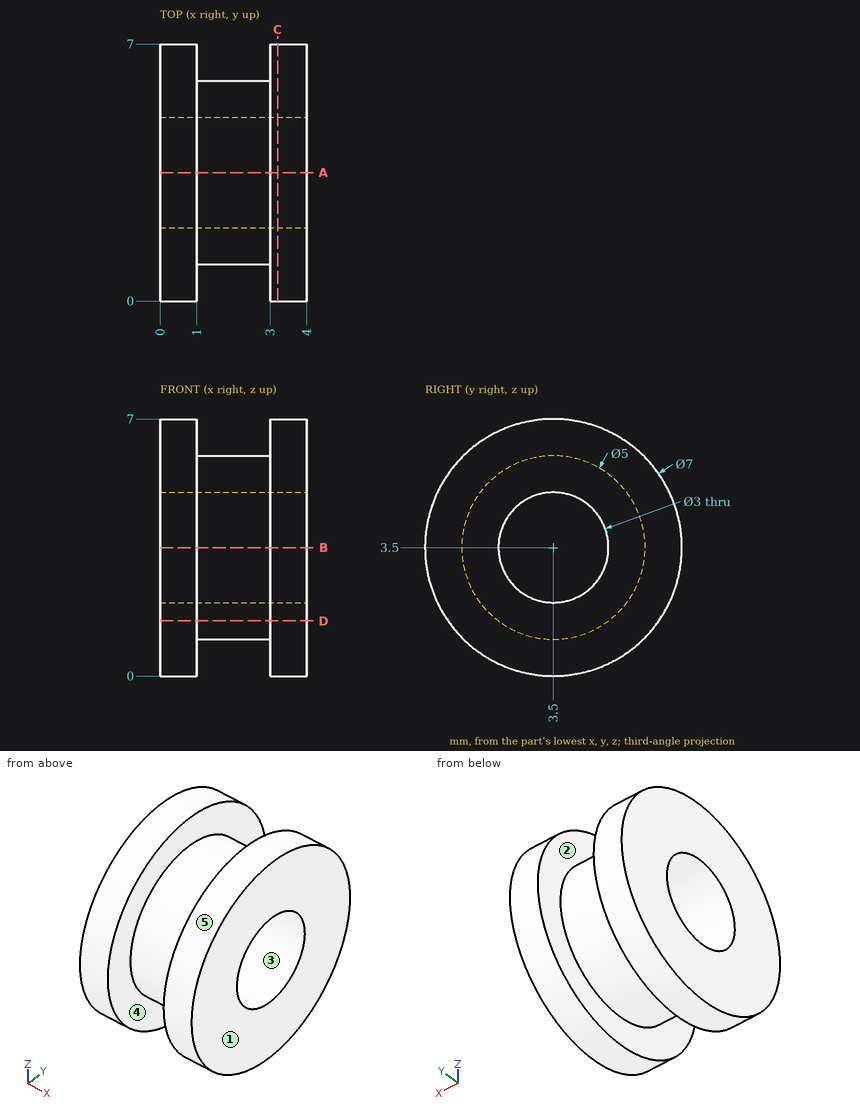
Job drawing, mm, ordinate dimensions from the low corner. One solid piece. A direction names the side the tool comes from. Give positions to 0.01 mm unless a question says otherwise; leave off trailing zeros. Loops run counter-clockwise (first coordinate to the right, second up) from the corner with the lowest first, then second, coordinate; pieces in that order, holes last.
Item 1: Slice it at A-A, the plane y = 3.5. List the corners of the cut face in (x, z).
Answers follow:
outline: (0, 0) - (1, 0) - (1, 1) - (3, 1) - (3, 0) - (4, 0) - (4, 2) - (0, 2) - close; (0, 5) - (4, 5) - (4, 7) - (3, 7) - (3, 6) - (1, 6) - (1, 7) - (0, 7) - close
Item 2: Slice it at D-D, the plane z = 1.5. List the corners of the cut face in (x, y), and give its area (3 significant figures).
Answers follow:
outline: (0, 0.63) - (1, 0.63) - (1, 2) - (3, 2) - (3, 0.63) - (4, 0.63) - (4, 6.37) - (3, 6.37) - (3, 5) - (1, 5) - (1, 6.37) - (0, 6.37) - close
area: 17.5 mm2
Item 3: Slice it at C-C, the plane x = 3.2. List the corners of the cut face in (y, z), and give its area (3 significant figures).
Answers follow:
outline: circle Ø7 at (3.5, 3.5); hole circle Ø3 at (3.5, 3.5)
area: 31.4 mm2
Item 4: Drill centre lines: line 1 (X direction, y = 6.5, z = 1.75); line 2 (Y direction, x = 1.55, z = 3.5); line 3 (Z direction, x = 2.6, y = 5.5). Where is each one in solid material? Low to high.
Answers follow:
line 1: x = 0 to 1, 3 to 4
line 2: y = 1 to 2, 5 to 6
line 3: z = 2 to 5
Item 5: Pull direction Y, two halves, no side cores. Call the marked faces 3, 4 and 5: released by +Y, released by -Y, zero draft, split by the parting line, or undercut.
Answers follow:
face 3: undercut
face 4: zero draft
face 5: split by the parting line
Item 6: Which spindle directions (+Z, -Z, +X, -X, +Y, -Y) get a long thin tool onto all of the face, cutting with end or side? Do the marked faces 1 and 2. Say none if no direction does.
Answers follow:
face 1: +Z, -Z, +X, +Y, -Y
face 2: none
